Input: part model. Units: mm. Frame: model coordinates. A direction names the side the tool comes from. Coordinates: 2 decimals unless noted, no trailing zeros. Write each loop counter-clockwise with the first axis right and the second up, starting at its lowest first coordinate (ties: lowest second). Pieces come first, ordered by that corner, then holes. Notation, with made-up numbers: (49.25, 76) -> (79.25, 76) arc R15 ccw to (79.25, 94) -> close; hole circle Ø8 at (75.25, 38.5). An arc over 180 degrees is marked (long way). Use one line per item in the form item = value. Start each with the question number.
(1) Set-up query: faces 4 (the face through (-12, 14.5, 17)), 5 (the face through (-17.001, -23, 3)), 6 (the face through (9, -10.5, 15)). Return all of +Z, -Z, +X, -X, +Y, -Y with unobstructed straight access to the full face (end or side cutting, diameter ignored); none if empty.
(2) First-contact query: pin 1 (1.5 mm diameter, centred on x = -2.5, z = 7.5, fed in from -Y); pin 2 (3 mm diameter, centred on y = 12, z = 19.5, fed in from -X); pin 3 (1 mm diameter, centred on y = -9.5, z = 15, fed in from +X); pin 4 (1.1 mm diameter, centred on x = 23, z = 3.5, fed in from -Y). Flat tips, straight axial feed; report the tip coordinate or a pass-through.
(3) Cut plane B-B on y = 0. Return the cut outline in (x, z).
(4) Ray query, line 1 along Y through (x, z) = (0, 1.65); line 2 along Y through (x, z) = (9, 19.5); line 3 along Z through (x, y) = (-16.5, 6.5). Return the intervals inside material, ascending.
(5) Pull-direction query (X, two-part tool) for faces 1 (the face through (23, 17.001, 3)), 2 (the face through (19.132, 19.193, 2.535)), 3 (the face through (8.5, 13, 16)); classes: released by +X, released by -X, zero draft, split by the parting line, or undercut.
(6) Cut plane D-D on z = 3.25. Return the cut outline in (x, y).
(7) Cut plane C-C on x = -6. Return the cut outline in (y, z), plus the area to 3 significant figures.
(8) Cut plane A-A on z = 17. Return the cut outline in (x, y), plus the area to 3 significant figures.
Autodesk Inventor part; units mm, degrees
ref_plane "YZ Plane" through (0, 0, 0) normal (1, 0, 0) x (0, 1, 0)
ref_plane "XZ Plane" through (0, 0, 0) normal (0, 1, 0) x (-1, 0, 0)
ref_plane "XY Plane" through (0, 0, 0) normal (0, 0, 1) x (1, 0, 0)
sketch "Sketch1" plane through (0, 0, 0) normal (0, 0, 1) x (1, 0, 0)
  line L0 (-34.86, 0) -> (34.86, 0) construction
  line L1 (0, -34.86) -> (0, 34.86) construction
  line L2 (0, 0) -> (16.9726, 16.9726) construction
  line L3 (0, 0) -> (24.0028, 0) construction
  line L4 (0, 24.9) -> (16.8009, 24.9)
  line L5 (16.8009, 24.9) -> (16.8009, 21.2415)
  line L6 (16.8009, 21.2415) -> (19.0212, 19.0212)
  line L7 (24.9, 0) -> (24.9, 16.8009)
  line L8 (24.9, 16.8009) -> (21.2415, 16.8009)
  line L9 (21.2415, 16.8009) -> (19.0212, 19.0212)
  line L10 (0, -24.9) -> (16.8009, -24.9)
  line L11 (16.8009, -24.9) -> (16.8009, -21.2415)
  line L12 (16.8009, -21.2415) -> (19.0212, -19.0212)
  line L13 (24.9, 0) -> (24.9, -16.8009)
  line L14 (24.9, -16.8009) -> (21.2415, -16.8009)
  line L15 (21.2415, -16.8009) -> (19.0212, -19.0212)
  line L16 (0, 0) -> (-16.9726, 16.9726) construction
  line L17 (0, 0) -> (-24.0028, 0) construction
  line L18 (0, 24.9) -> (-16.8009, 24.9)
  line L19 (-16.8009, 24.9) -> (-16.8009, 21.2415)
  line L20 (-16.8009, 21.2415) -> (-19.0212, 19.0212)
  line L21 (-24.9, 0) -> (-24.9, 16.8009)
  line L22 (-24.9, 16.8009) -> (-21.2415, 16.8009)
  line L23 (-21.2415, 16.8009) -> (-19.0212, 19.0212)
  line L24 (0, -24.9) -> (-16.8009, -24.9)
  line L25 (-16.8009, -24.9) -> (-16.8009, -21.2415)
  line L26 (-16.8009, -21.2415) -> (-19.0212, -19.0212)
  line L27 (-21.2415, -16.8009) -> (-19.0212, -19.0212)
  line L28 (-24.9, -16.8009) -> (-21.2415, -16.8009)
  line L29 (-24.9, 0) -> (-24.9, -16.8009)
  circle A0 centre (0, 0) radius 10
  dimension "d17" = 45
  dimension "d18" = 24.9
  dimension "d20" = 3.14
  dimension "d21" = 26.9
  dimension "d22" = 20
extrude "Extrusion1" add sketch "Sketch1" along normal blind 5
sketch "Skizze6" plane through (0, 0, 5) normal (0, 0, 1) x (1, 0, 0)
  circle A0 centre (0, 0) radius 10 construction
  line L0 (16.8009, 24.9) -> (-16.8009, 24.9) construction
  line L1 (-16.8009, 24.9) -> (-16.8009, 21.2415)
  line L2 (-16.8009, 21.2415) -> (-21.2415, 16.8009)
  line L3 (-21.2415, 16.8009) -> (-24.9, 16.8009)
  line L4 (-24.9, 16.8009) -> (-24.9, -16.8009) construction
  line L5 (-24.9, -16.8009) -> (-21.2415, -16.8009)
  line L6 (-21.2415, -16.8009) -> (-16.8009, -21.2415)
  line L7 (-16.8009, -21.2415) -> (-16.8009, -24.9)
  line L8 (-16.8009, -24.9) -> (16.8009, -24.9) construction
  line L9 (16.8009, -24.9) -> (16.8009, -21.2415)
  line L10 (16.8009, -21.2415) -> (21.2415, -16.8009)
  line L11 (21.2415, -16.8009) -> (24.9, -16.8009)
  line L12 (24.9, -16.8009) -> (24.9, 16.8009) construction
  line L13 (24.9, 16.8009) -> (21.2415, 16.8009)
  line L14 (21.2415, 16.8009) -> (16.8009, 21.2415)
  line L15 (16.8009, 21.2415) -> (16.8009, 24.9)
  line L16 (-17.0009, 25.1) -> (17.0009, 25.1) construction
  line L17 (17.0009, 25.1) -> (17.0009, 21.3243)
  line L18 (17.0009, 21.3243) -> (21.3243, 17.0009)
  line L19 (21.3243, 17.0009) -> (25.1, 17.0009)
  line L20 (25.1, 17.0009) -> (25.1, -17.0009) construction
  line L21 (25.1, -17.0009) -> (21.3243, -17.0009)
  line L22 (21.3243, -17.0009) -> (17.0009, -21.3243)
  line L23 (17.0009, -21.3243) -> (17.0009, -25.1)
  line L24 (17.0009, -25.1) -> (-17.0009, -25.1) construction
  line L25 (-17.0009, -25.1) -> (-17.0009, -21.3243)
  line L26 (-17.0009, -21.3243) -> (-21.3243, -17.0009)
  line L27 (-21.3243, -17.0009) -> (-25.1, -17.0009)
  line L28 (-25.1, -17.0009) -> (-25.1, 17.0009) construction
  line L29 (-25.1, 17.0009) -> (-21.3243, 17.0009)
  line L30 (-21.3243, 17.0009) -> (-17.0009, 21.3243)
  line L31 (-17.0009, 21.3243) -> (-17.0009, 25.1)
  line L32 (-24.9, 16.8009) -> (-24.9, 17.0009)
  line L33 (-16.8009, 24.9) -> (-17.0009, 24.9)
  line L34 (16.8009, 24.9) -> (-16.8009, 24.9)
  line L35 (16.8009, 24.9) -> (17.0009, 24.9)
  line L36 (24.9, 16.8009) -> (24.9, 17.0009)
  line L37 (16.8009, -24.9) -> (17.0009, -24.9)
  line L38 (21.2415, -16.8009) -> (24.9, -16.8009)
  line L39 (24.9, -16.8009) -> (24.9, -17.0009)
  line L40 (-16.8009, -24.9) -> (-17.0009, -24.9)
  line L41 (-24.9, -16.8009) -> (-21.2415, -16.8009)
  line L42 (-24.9, -16.8009) -> (-24.9, -17.0009)
  dimension "d17" = 45
  dimension "d18" = 24.9
  dimension "d20" = 3.14
  dimension "d21" = 26.9
  dimension "d41" = 0.2
extrude "IM_offset" add sketch "Skizze6" against normal up to surface (5 mm away)
sketch "Sketch8" plane through (0, 0, 5) normal (0, 0, 1) x (1, 0, 0)
  circle A0 centre (0, 0) radius 10
  line L0 (-10.5, -10.5) -> (10.5, -10.5)
  line L1 (10.5, -10.5) -> (10.5, 10.5)
  line L2 (10.5, 10.5) -> (-10.5, 10.5)
  line L3 (-10.5, 10.5) -> (-10.5, -10.5)
  line L4 (-10.5, -10.5) -> (10.5, 10.5) construction
  line L5 (10.5, -10.5) -> (-10.5, 10.5) construction
  line L6 (-10.5, -10.5) -> (10.5, -10.5) construction
  line L7 (14.5, 14.5) -> (14.5, -14.5)
  line L8 (14.5, -14.5) -> (-14.5, -14.5)
  line L9 (-14.5, -14.5) -> (-14.5, 14.5)
  line L10 (-14.5, 14.5) -> (14.5, 14.5)
  dimension "d48" = 21
  dimension "d49" = 0
  dimension "d50" = 21
  dimension "d51" = 4
extrude "Extrusion8" add sketch "Sketch8" along normal blind 21 contours L7 L8 L9 L10
sketch "Sketch9" plane through (0, 0, 26) normal (0, 0, 1) x (1, 0, 0)
  line L0 (17.0009, 24.9) -> (-17.0009, 24.9)
  line L1 (-17.0009, 24.9) -> (-17.0009, 21.3243)
  line L2 (-17.0009, 21.3243) -> (-21.3243, 17.0009)
  line L3 (-21.3243, 17.0009) -> (-24.9, 17.0009)
  line L4 (-24.9, 17.0009) -> (-24.9, -17.0009)
  line L5 (-24.9, -17.0009) -> (-21.3243, -17.0009)
  line L6 (-21.3243, -17.0009) -> (-17.0009, -21.3243)
  line L7 (-17.0009, -21.3243) -> (-17.0009, -24.9)
  line L8 (-17.0009, -24.9) -> (17.0009, -24.9)
  line L9 (17.0009, -24.9) -> (17.0009, -21.3243)
  line L10 (17.0009, -21.3243) -> (21.3243, -17.0009)
  line L11 (21.3243, -17.0009) -> (24.9, -17.0009)
  line L12 (24.9, -17.0009) -> (24.9, 17.0009)
  line L13 (24.9, 17.0009) -> (21.3243, 17.0009)
  line L14 (21.3243, 17.0009) -> (17.0009, 21.3243)
  line L15 (17.0009, 21.3243) -> (17.0009, 24.9)
  line L16 (-14.5, 14.5) -> (14.5, 14.5)
  line L17 (14.5, 14.5) -> (14.5, -14.5)
  line L18 (14.5, -14.5) -> (-14.5, -14.5)
  line L19 (-14.5, -14.5) -> (-14.5, 14.5)
  line L20 (24.9, -8.5) -> (-24.9, -8.5)
  line L21 (-24.9, -8.5) -> (-24.9, 8.5)
  line L22 (-24.9, 8.5) -> (24.9, 8.5)
  line L23 (24.9, 8.5) -> (24.9, -8.5)
  line L24 (24.9, -8.5) -> (-24.9, 8.5) construction
  line L25 (-24.9, -8.5) -> (24.9, 8.5) construction
  line L26 (8.5, -24.9) -> (8.5, 24.9)
  line L27 (8.5, 24.9) -> (-8.5, 24.9)
  line L28 (-8.5, 24.9) -> (-8.5, -24.9)
  line L29 (-8.5, -24.9) -> (8.5, -24.9)
  line L30 (8.5, -24.9) -> (-8.5, 24.9) construction
  line L31 (8.5, 24.9) -> (-8.5, -24.9) construction
  point P0 (0, 0)
  point P1 (-8.5, -8.5)
  point P2 (8.5, -8.5)
  point P3 (8.5, 8.5)
  point P4 (-8.5, 8.5)
  dimension "d54" = 17
  dimension "d55" = 17
extrude "Extrusion9" cut sketch "Sketch9" against normal blind 21 contours L26 L16 L28 L0 | L26 L22 L28 L16 | L26 L20 L28 L22 | L22 L17 L20 L26 | L28 L20 L19 L22 | L22 L12 L20 L17 | L26 L18 L28 L20 | L19 L20 L4 L22 | L26 L8 L28 L18
chamfer "Chamfer1" distance 4 angle 45 8 edges at (-11.5, 14.5, 5) (11.5, 14.5, 5) (-14.5, 11.5, 5) (-14.5, -11.5, 5) (-11.5, -14.5, 5) (11.5, -14.5, 5) (14.5, -11.5, 5) (14.5, 11.5, 5)
properties part number "20_Cube_Insert_Beamsplitter_v3"
Values:
q1.face_4 = +Z, +X, -X, +Y
q1.face_5 = +Z, -Z, -X, -Y
q1.face_6 = +Z
q2.pin_1 = through
q2.pin_2 = -14.5
q2.pin_3 = 14.5
q2.pin_4 = -17
q3.outline = (-24.9, 0) -> (-10, 0) -> (-10, 5) -> (-24.9, 5) -> close; (10, 0) -> (24.9, 0) -> (24.9, 5) -> (10, 5) -> close
q4.line_1 = -24.9 to -10, 10 to 24.9
q4.line_2 = -14.5 to -10.5, 10.5 to 14.5
q4.line_3 = 0 to 5
q5.face_1 = zero draft
q5.face_2 = released by +X
q5.face_3 = undercut
q6.outline = (-24.9, -17) -> (-21.32, -17) -> (-17, -21.32) -> (-17, -24.9) -> (17, -24.9) -> (17, -21.32) -> (21.32, -17) -> (24.9, -17) -> (24.9, 17) -> (21.32, 17) -> (17, 21.32) -> (17, 24.9) -> (-17, 24.9) -> (-17, 21.32) -> (-21.32, 17) -> (-24.9, 17) -> close; hole circle Ø20 at (0, 0)
q7.outline = (-24.9, 0) -> (-8, 0) -> (-8, 5) -> (-24.9, 5) -> close; (8, 0) -> (24.9, 0) -> (24.9, 5) -> (8, 5) -> close
q7.area = 169 mm2
q8.outline = (-14.5, -14.5) -> (-8.5, -14.5) -> (-8.5, -10.5) -> (-10.5, -10.5) -> (-10.5, -8.5) -> (-14.5, -8.5) -> close; (-14.5, 8.5) -> (-10.5, 8.5) -> (-10.5, 10.5) -> (-8.5, 10.5) -> (-8.5, 14.5) -> (-14.5, 14.5) -> close; (8.5, -14.5) -> (14.5, -14.5) -> (14.5, -8.5) -> (10.5, -8.5) -> (10.5, -10.5) -> (8.5, -10.5) -> close; (8.5, 10.5) -> (10.5, 10.5) -> (10.5, 8.5) -> (14.5, 8.5) -> (14.5, 14.5) -> (8.5, 14.5) -> close
q8.area = 128 mm2
